from build123d import *

# Parameters (mm, degrees)
BOSS_EXTRUDE1_DEPTH      = 2.413
BOSS_EXTRUDE2_DEPTH      = 8.382
BOSS_EXTRUDE2_DEPTH_BACK = 28.448
SKETCH3_W                = 42.545
SKETCH3_H                = 19.685
BOSS_EXTRUDE3_DEPTH      = 2.54
SKETCH5_R                = 6.5405
BOSS_EXTRUDE4_DEPTH      = 1.905
SKETCH6_R                = 2.9845
BOSS_EXTRUDE5_DEPTH      = 4.191


with BuildPart() as part:
    # Sketch2 → Boss-Extrude1 (new body)
    with BuildSketch(Plane(origin=(0, 0, 0), x_dir=(1, 0, 0), z_dir=(0, 1, 0))):
        with BuildLine():
            Line((-27.051, -9.8425), (27.051, -9.8425))
            Line((27.051, -9.8425), (27.051, -5.7785))
            Line((27.051, -5.7785), (26.416, -5.7785))
            ThreePointArc((26.416, -5.7785), (22.352, -4.7625), (26.416, -3.7465))
            Line((26.416, -3.7465), (27.051, -3.7465))
            Line((27.051, -3.7465), (27.051, 3.7465))
            Line((27.051, 3.7465), (26.416, 3.7465))
            ThreePointArc((26.416, 3.7465), (22.352, 4.7625), (26.416, 5.7785))
            Line((26.416, 5.7785), (27.051, 5.7785))
            Line((27.051, 5.7785), (27.051, 9.8425))
            Line((27.051, 9.8425), (-27.051, 9.8425))
            Line((-27.051, 9.8425), (-27.051, 5.7785))
            Line((-27.051, 5.7785), (-26.416, 5.7785))
            ThreePointArc((-26.416, 5.7785), (-22.352, 4.7625), (-26.416, 3.7465))
            Line((-26.416, 3.7465), (-27.051, 3.7465))
            Line((-27.051, 3.7465), (-27.051, -3.7465))
            Line((-27.051, -3.7465), (-26.416, -3.7465))
            ThreePointArc((-26.416, -3.7465), (-22.352, -4.7625), (-26.416, -5.7785))
            Line((-26.416, -5.7785), (-27.051, -5.7785))
            Line((-27.051, -5.7785), (-27.051, -9.8425))
        make_face()
    extrude(amount=BOSS_EXTRUDE1_DEPTH)

    # Sketch3 → Boss-Extrude2 (add, two sides: drawn at the far end of the back side and taken through both)
    with BuildSketch(Plane(origin=(0, 0, 0), x_dir=(1, 0, 0), z_dir=(0, 1, 0)).offset(-BOSS_EXTRUDE2_DEPTH_BACK)):
        Rectangle(SKETCH3_W, SKETCH3_H)
    extrude(amount=BOSS_EXTRUDE2_DEPTH + BOSS_EXTRUDE2_DEPTH_BACK)

    # Sketch4 → Boss-Extrude3 (add)
    with BuildSketch(Plane(origin=(0, 8.382, 0), x_dir=(1, 0, 0), z_dir=(0, 1, 0))):
        with BuildLine():
            Line((-15.6845, 8.9535), (7.342256857, 8.9535))
            ThreePointArc((7.342256857, 8.9535), (21.2725, 0), (7.342256857, -8.9535))
            Line((7.342256857, -8.9535), (-15.6845, -8.9535))
            Line((-15.6845, -8.9535), (-15.6845, 8.9535))
        make_face()
    extrude(amount=BOSS_EXTRUDE3_DEPTH)

    # Sketch5 → Boss-Extrude4 (add)
    with BuildSketch(Plane(origin=(0, 10.922, 0), x_dir=(1, 0, 0), z_dir=(0, 1, 0))):
        with Locations(Location((11.43, 0, 0), (0, 0, 90))):
            Circle(SKETCH5_R)
    extrude(amount=BOSS_EXTRUDE4_DEPTH)

    # Sketch6 → Boss-Extrude5 (add)
    with BuildSketch(Plane(origin=(0, 12.827, 0), x_dir=(1, 0, 0), z_dir=(0, 1, 0))):
        with Locations(Location((11.43, 0, 0), (0, 0, 270))):
            Circle(SKETCH6_R)
    extrude(amount=BOSS_EXTRUDE5_DEPTH)


solid = part.part
Model file for the job. Use its own axes, mm. A direction names the side the tool comes from. Give positions to 0.01 mm unless a question says otherwise; leave off trailing zeros. Loops run counter-clockwise (first coordinate to the right, second up) from the corner with the lowest first, then second, coordinate; pieces in that order, holes last. Notation, with made-up numbers: (46, -30) -> (76, -30) arc R22 ccw to (76, -12) -> close; hole circle Ø6 at (63, 11). An arc over 180 degrees is marked (long way). Use a Markdown table: item, result. Add a question column.
(1) Wall check: line 1 along X through (y, z) = (-1.5, -4.25); line 2 along Y through (x, z) = (16.5, 5.25); line 3 along Y through (x, z) = (-18, -1.25). Give the ranges that are in metal, low to high.
(2) Slice it at B-B on x = -23. List the corners of the cut face in (y, z), and give its area (3 significant figures).
(3) Slice it at C-C on z = -1.5. List the corners of the cut face in (x, y), and give its area (3 significant figures).
(4) Slice it at A-A on x = 4. List the corners of the cut face in (y, z).
(5) Tool access for faces 1 (the cylindrical face through (21.27, 9.63, -0.28)), 2 (the flat face through (-4, 10, 8.954)), 3 (the flat face through (-21.272, -14, 0)), 4 (the flat face through (-24, 2.413, 0)): list every direction of +Z, -Z, +X, -X, +Y, -Y with a clear straight run to the whole face (end or side of a thin tool).
(6) Slice it at D-D on y = 12. List the corners of the cut face in (x, z), and give its area (3 significant figures).
(7) Drop flat-ended pins along their axis: pin 1 Ø11 at (x, z) = (14, -6.5) entering from +Y; pin 2 Ø3 at (y, z) = (9.5, 0.5) entering from -X; pin 3 Ø1.7 at (x, z) = (23, 3.5) entering from +Y; pin 4 Ø3 at (x, y) = (-8.5, 10) entering from -Z. Give the stop position or say it passes through.
Filled sheet:
| question | item | result |
|---|---|---|
| 1 | line 1 | -21.27 to 21.27 |
| 1 | line 2 | -28.45 to 10.92 |
| 1 | line 3 | -28.45 to 8.38 |
| 2 | outline | (0, -9.84) -> (2.41, -9.84) -> (2.41, -6.3) -> (0, -6.3) -> close; (0, -3.22) -> (2.41, -3.22) -> (2.41, 3.22) -> (0, 3.22) -> close; (0, 6.3) -> (2.41, 6.3) -> (2.41, 9.84) -> (0, 9.84) -> close |
| 2 | area | 32.6 mm2 |
| 3 | outline | (-27.05, 0) -> (-21.27, 0) -> (-21.27, -28.45) -> (21.27, -28.45) -> (21.27, 0) -> (27.05, 0) -> (27.05, 2.41) -> (21.27, 2.41) -> (21.27, 8.38) -> (21.16, 8.38) -> (21.16, 10.92) -> (17.8, 10.92) -> (17.8, 12.83) -> (14.01, 12.83) -> (14.01, 17.02) -> (8.85, 17.02) -> (8.85, 12.83) -> (5.06, 12.83) -> (5.06, 10.92) -> (-15.68, 10.92) -> (-15.68, 8.38) -> (-21.27, 8.38) -> (-21.27, 2.41) -> (-27.05, 2.41) -> close |
| 3 | area | 1,730 mm2 |
| 4 | outline | (-28.45, -9.84) -> (8.38, -9.84) -> (8.38, -8.95) -> (10.92, -8.95) -> (10.92, 8.95) -> (8.38, 8.95) -> (8.38, 9.84) -> (-28.45, 9.84) -> close |
| 5 | face 1 | +Y |
| 5 | face 2 | +Z, -X, +Y |
| 5 | face 3 | +Z, -Z, -X, -Y |
| 5 | face 4 | +Z, -Z, -X, +Y |
| 6 | outline | circle Ø13.08 at (11.43, 0) |
| 6 | area | 134 mm2 |
| 7 | pin 1 | y = 17.02 |
| 7 | pin 2 | x = -21.27 |
| 7 | pin 3 | y = 2.41 |
| 7 | pin 4 | z = -8.95 |
